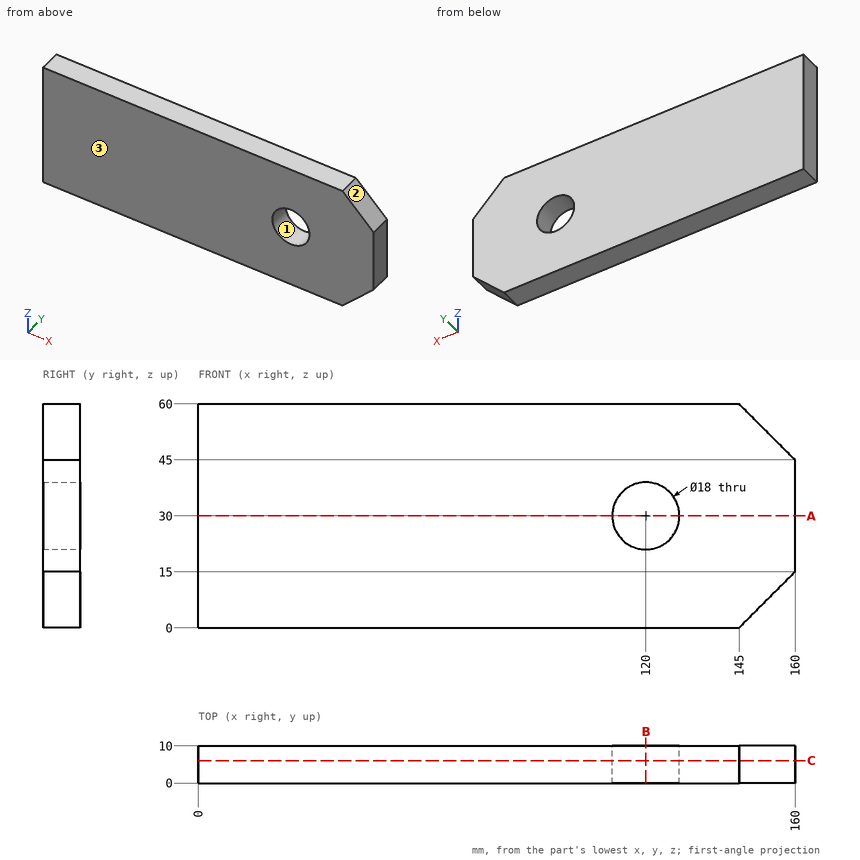
Source: three-view drawing plus pictorial views. Frame: mm from the lowest corner of the part. Round coordinates to 2 decimals unless told otherwise and drop trailing zeros. Order: outer loops, then holes, each group sorted by start corner. A loop starts at its lowest first (then second) coordinate and runs counter-clockwise, first axis right, second up. Notation, with made-up numbers: (5.5, 43.25) -> (43.5, 43.25) arc R16 cw to (43.5, 59.25) -> close; hole circle Ø8 at (17.25, -6). An arc over 180 degrees is marked (long way). Use one line per item in the form item = value.
(1) Section C-C on y = 6. Return loops of the section in (x, z).
Results list:
outline = (0, 0) -> (145, 0) -> (160, 15) -> (160, 45) -> (145, 60) -> (0, 60) -> close; hole circle Ø18 at (120, 30)
(2) Ray query, probe 1 along Z at (x, y) = (120, 4.5); probe 2 along X at (y, z) = (6.25, 12.5); probe 3 along X at (y, z) = (1.25, 49.5). Return the intervals inside material, ascending. Write a range as [from, to].
Results list:
probe_1 = [0, 21], [39, 60]
probe_2 = [0, 157.5]
probe_3 = [0, 155.5]
(3) Draft query along Z for the marked faces 1, 2 and 3. Return one class per face: pulls with the +Z half, pulls with the -Z half, needs draft (parallel to the pull), parting line crosses it, or undercut.
Results list:
face_1 = undercut
face_2 = pulls with the +Z half
face_3 = needs draft
(4) Section A-A on z = 30. Return loops of the section in (x, y), and give its area (3 significant figures).
Results list:
outline = (0, 0) -> (111, 0) -> (111, 10) -> (0, 10) -> close; (129, 0) -> (160, 0) -> (160, 10) -> (129, 10) -> close
area = 1,420 mm^2
(5) Section B-B on x = 120. Return loops of the section in (y, z), and give its area (3 significant figures).
Results list:
outline = (0, 0) -> (10, 0) -> (10, 21) -> (0, 21) -> close; (0, 39) -> (10, 39) -> (10, 60) -> (0, 60) -> close
area = 420 mm^2
